```python
from build123d import *

# Parameters (mm, degrees)
SKETCH1_W            = 5
SKETCH1_H            = 4.25
SKETCH2_R            = 2.5
BOSS_EXTRUDE1_DEPTH  = 2.088407645
SKETCH3_R            = 2.5
BOSS_EXTRUDE2_DEPTH  = 0.311592355
BOSS_EXTRUDE2_TAPER  = 55
SKETCH4_R            = 2.055
BOSS_EXTRUDE3_DEPTH  = 0.311592355
BOSS_EXTRUDE3_TAPER  = -55
SKETCH5_R            = 2.5
BOSS_EXTRUDE4_DEPTH  = 0.136815291
SKETCH6_R            = 2.5
BOSS_EXTRUDE5_DEPTH  = 0.311592355
BOSS_EXTRUDE5_TAPER  = 55
SKETCH7_R            = 2.055
BOSS_EXTRUDE6_DEPTH  = 0.311592355
BOSS_EXTRUDE6_TAPER  = -55
SKETCH8_R            = 2.5
BOSS_EXTRUDE7_DEPTH  = 0.136815291
SKETCH9_R            = 2.5
BOSS_EXTRUDE8_DEPTH  = 0.311592355
BOSS_EXTRUDE8_TAPER  = 55
SKETCH10_R           = 2.055
BOSS_EXTRUDE9_DEPTH  = 0.311592355
BOSS_EXTRUDE9_TAPER  = -55
SKETCH11_R           = 2.5
BOSS_EXTRUDE10_DEPTH = 0.136815291
SKETCH12_R           = 2.5
BOSS_EXTRUDE11_DEPTH = 0.311592355
BOSS_EXTRUDE11_TAPER = 55
SKETCH13_R           = 2.055
BOSS_EXTRUDE12_DEPTH = 0.311592355
BOSS_EXTRUDE12_TAPER = -55
SKETCH14_R           = 2.5
BOSS_EXTRUDE13_DEPTH = 0.136815291
SKETCH15_R           = 2.5
BOSS_EXTRUDE14_DEPTH = 0.311592355
BOSS_EXTRUDE14_TAPER = 55
SKETCH16_R           = 2.055
BOSS_EXTRUDE15_DEPTH = 0.311592355
BOSS_EXTRUDE15_TAPER = -55
SKETCH17_R           = 2.5
BOSS_EXTRUDE16_DEPTH = 0.136815291
SKETCH18_R           = 2.5
BOSS_EXTRUDE17_DEPTH = 0.311592355
BOSS_EXTRUDE17_TAPER = 55
SKETCH19_R           = 2.055
BOSS_EXTRUDE18_DEPTH = 0.311592355
BOSS_EXTRUDE18_TAPER = -55
SKETCH20_R           = 2.5
BOSS_EXTRUDE19_DEPTH = 0.136815291
SKETCH21_R           = 2.5
BOSS_EXTRUDE20_DEPTH = 0.311592355
BOSS_EXTRUDE20_TAPER = 55
SKETCH22_R           = 2.055
BOSS_EXTRUDE21_DEPTH = 0.311592355
BOSS_EXTRUDE21_TAPER = -55
SKETCH23_R           = 2.5
BOSS_EXTRUDE22_DEPTH = 0.136815291
SKETCH24_R           = 2.5
BOSS_EXTRUDE23_DEPTH = 0.311592355
BOSS_EXTRUDE23_TAPER = 55
SKETCH25_R           = 2.055
BOSS_EXTRUDE24_DEPTH = 0.311592355
BOSS_EXTRUDE24_TAPER = -55
SKETCH26_R           = 2.5
BOSS_EXTRUDE25_DEPTH = 0.136815291
SKETCH27_R           = 2.5
BOSS_EXTRUDE26_DEPTH = 0.311592355
BOSS_EXTRUDE26_TAPER = 55
SKETCH28_R           = 2.055
BOSS_EXTRUDE27_DEPTH = 0.311592355
BOSS_EXTRUDE27_TAPER = -55
SKETCH29_R           = 2.5
BOSS_EXTRUDE28_DEPTH = 0.136815291
SKETCH30_R           = 2.5
BOSS_EXTRUDE29_DEPTH = 0.311592355
BOSS_EXTRUDE29_TAPER = 55
SKETCH31_R           = 2.055
BOSS_EXTRUDE30_DEPTH = 0.311592355
BOSS_EXTRUDE30_TAPER = -55
SKETCH32_R           = 2.5
BOSS_EXTRUDE31_DEPTH = 0.003407645
SKETCH33_R           = 2.5
BOSS_EXTRUDE32_DEPTH = 0.445
BOSS_EXTRUDE32_TAPER = 45
CUT_EXTRUDE1_DEPTH   = 2.5
FILLET1_R            = 0.2


with BuildPart() as part:
    # Sketch1 → Revolve1 (revolve)
    with BuildSketch(Plane(origin=(0, 0, 0), x_dir=(-1, 0, 0), z_dir=(0, 0, -1))):
        with Locations((6.290592114, 2.355818515)):
            Rectangle(SKETCH1_W, SKETCH1_H)
    revolve(axis=Axis((-3.790592114, 0.230818515, 0), (-1, 0, 0)))

    # Sketch2 → Boss-Extrude1 (add)
    with BuildSketch(Plane(origin=(-3.790592114, 0, 0), x_dir=(0, 0, -1), z_dir=(1, 0, 0))):
        with Locations((0, 0.230818515)):
            Circle(SKETCH2_R)
    extrude(amount=BOSS_EXTRUDE1_DEPTH)

    # Sketch3 → Boss-Extrude2 (add)
    with BuildSketch(Plane(origin=(-1.702184469, 0, 0), x_dir=(0, 0, -1), z_dir=(1, 0, 0))):
        with Locations((0, 0.230818515)):
            Circle(SKETCH3_R)
    extrude(amount=BOSS_EXTRUDE2_DEPTH, taper=BOSS_EXTRUDE2_TAPER)

    # Sketch4 → Boss-Extrude3 (add)
    with BuildSketch(Plane(origin=(-1.390592114, 0, 0), x_dir=(0, 0, -1), z_dir=(1, 0, 0))):
        with Locations((0, 0.230818515)):
            Circle(SKETCH4_R)
    extrude(amount=BOSS_EXTRUDE3_DEPTH, taper=BOSS_EXTRUDE3_TAPER)

    # Sketch5 → Boss-Extrude4 (add)
    with BuildSketch(Plane(origin=(-1.07899976, 0, 0), x_dir=(0, 0, -1), z_dir=(1, 0, 0))):
        with Locations((0, 0.230818515)):
            Circle(SKETCH5_R)
    extrude(amount=BOSS_EXTRUDE4_DEPTH)

    # Sketch6 → Boss-Extrude5 (add)
    with BuildSketch(Plane(origin=(-0.942184469, 0, 0), x_dir=(0, 0, -1), z_dir=(1, 0, 0))):
        with Locations((0, 0.230818515)):
            Circle(SKETCH6_R)
    extrude(amount=BOSS_EXTRUDE5_DEPTH, taper=BOSS_EXTRUDE5_TAPER)

    # Sketch7 → Boss-Extrude6 (add)
    with BuildSketch(Plane(origin=(-0.630592114, 0, 0), x_dir=(0, 0, -1), z_dir=(1, 0, 0))):
        with Locations((0, 0.230818515)):
            Circle(SKETCH7_R)
    extrude(amount=BOSS_EXTRUDE6_DEPTH, taper=BOSS_EXTRUDE6_TAPER)

    # Sketch8 → Boss-Extrude7 (add)
    with BuildSketch(Plane(origin=(-0.31899976, 0, 0), x_dir=(0, 0, -1), z_dir=(1, 0, 0))):
        with Locations((0, 0.230818515)):
            Circle(SKETCH8_R)
    extrude(amount=BOSS_EXTRUDE7_DEPTH)

    # Sketch9 → Boss-Extrude8 (add)
    with BuildSketch(Plane(origin=(-0.182184469, 0, 0), x_dir=(0, 0, -1), z_dir=(1, 0, 0))):
        with Locations((0, 0.230818515)):
            Circle(SKETCH9_R)
    extrude(amount=BOSS_EXTRUDE8_DEPTH, taper=BOSS_EXTRUDE8_TAPER)

    # Sketch10 → Boss-Extrude9 (add)
    with BuildSketch(Plane(origin=(0.129407886, 0, 0), x_dir=(0, 0, -1), z_dir=(1, 0, 0))):
        with Locations((0, 0.230818515)):
            Circle(SKETCH10_R)
    extrude(amount=BOSS_EXTRUDE9_DEPTH, taper=BOSS_EXTRUDE9_TAPER)

    # Sketch11 → Boss-Extrude10 (add)
    with BuildSketch(Plane(origin=(0.44100024, 0, 0), x_dir=(0, 0, -1), z_dir=(1, 0, 0))):
        with Locations((0, 0.230818515)):
            Circle(SKETCH11_R)
    extrude(amount=BOSS_EXTRUDE10_DEPTH)

    # Sketch12 → Boss-Extrude11 (add)
    with BuildSketch(Plane(origin=(0.577815531, 0, 0), x_dir=(0, 0, -1), z_dir=(1, 0, 0))):
        with Locations((0, 0.230818515)):
            Circle(SKETCH12_R)
    extrude(amount=BOSS_EXTRUDE11_DEPTH, taper=BOSS_EXTRUDE11_TAPER)

    # Sketch13 → Boss-Extrude12 (add)
    with BuildSketch(Plane(origin=(0.889407886, 0, 0), x_dir=(0, 0, -1), z_dir=(1, 0, 0))):
        with Locations((0, 0.230818515)):
            Circle(SKETCH13_R)
    extrude(amount=BOSS_EXTRUDE12_DEPTH, taper=BOSS_EXTRUDE12_TAPER)

    # Sketch14 → Boss-Extrude13 (add)
    with BuildSketch(Plane(origin=(1.20100024, 0, 0), x_dir=(0, 0, -1), z_dir=(1, 0, 0))):
        with Locations((0, 0.230818515)):
            Circle(SKETCH14_R)
    extrude(amount=BOSS_EXTRUDE13_DEPTH)

    # Sketch15 → Boss-Extrude14 (add)
    with BuildSketch(Plane(origin=(1.337815531, 0, 0), x_dir=(0, 0, -1), z_dir=(1, 0, 0))):
        with Locations((0, 0.230818515)):
            Circle(SKETCH15_R)
    extrude(amount=BOSS_EXTRUDE14_DEPTH, taper=BOSS_EXTRUDE14_TAPER)

    # Sketch16 → Boss-Extrude15 (add)
    with BuildSketch(Plane(origin=(1.649407886, 0, 0), x_dir=(0, 0, -1), z_dir=(1, 0, 0))):
        with Locations((0, 0.230818515)):
            Circle(SKETCH16_R)
    extrude(amount=BOSS_EXTRUDE15_DEPTH, taper=BOSS_EXTRUDE15_TAPER)

    # Sketch17 → Boss-Extrude16 (add)
    with BuildSketch(Plane(origin=(1.96100024, 0, 0), x_dir=(0, 0, -1), z_dir=(1, 0, 0))):
        with Locations((0, 0.230818515)):
            Circle(SKETCH17_R)
    extrude(amount=BOSS_EXTRUDE16_DEPTH)

    # Sketch18 → Boss-Extrude17 (add)
    with BuildSketch(Plane(origin=(2.097815531, 0, 0), x_dir=(0, 0, -1), z_dir=(1, 0, 0))):
        with Locations((0, 0.230818515)):
            Circle(SKETCH18_R)
    extrude(amount=BOSS_EXTRUDE17_DEPTH, taper=BOSS_EXTRUDE17_TAPER)

    # Sketch19 → Boss-Extrude18 (add)
    with BuildSketch(Plane(origin=(2.409407886, 0, 0), x_dir=(0, 0, -1), z_dir=(1, 0, 0))):
        with Locations((0, 0.230818515)):
            Circle(SKETCH19_R)
    extrude(amount=BOSS_EXTRUDE18_DEPTH, taper=BOSS_EXTRUDE18_TAPER)

    # Sketch20 → Boss-Extrude19 (add)
    with BuildSketch(Plane(origin=(2.72100024, 0, 0), x_dir=(0, 0, -1), z_dir=(1, 0, 0))):
        with Locations((0, 0.230818515)):
            Circle(SKETCH20_R)
    extrude(amount=BOSS_EXTRUDE19_DEPTH)

    # Sketch21 → Boss-Extrude20 (add)
    with BuildSketch(Plane(origin=(2.857815531, 0, 0), x_dir=(0, 0, -1), z_dir=(1, 0, 0))):
        with Locations((0, 0.230818515)):
            Circle(SKETCH21_R)
    extrude(amount=BOSS_EXTRUDE20_DEPTH, taper=BOSS_EXTRUDE20_TAPER)

    # Sketch22 → Boss-Extrude21 (add)
    with BuildSketch(Plane(origin=(3.169407886, 0, 0), x_dir=(0, 0, -1), z_dir=(1, 0, 0))):
        with Locations((0, 0.230818515)):
            Circle(SKETCH22_R)
    extrude(amount=BOSS_EXTRUDE21_DEPTH, taper=BOSS_EXTRUDE21_TAPER)

    # Sketch23 → Boss-Extrude22 (add)
    with BuildSketch(Plane(origin=(3.48100024, 0, 0), x_dir=(0, 0, -1), z_dir=(1, 0, 0))):
        with Locations((0, 0.230818515)):
            Circle(SKETCH23_R)
    extrude(amount=BOSS_EXTRUDE22_DEPTH)

    # Sketch24 → Boss-Extrude23 (add)
    with BuildSketch(Plane(origin=(3.617815531, 0, 0), x_dir=(0, 0, -1), z_dir=(1, 0, 0))):
        with Locations((0, 0.230818515)):
            Circle(SKETCH24_R)
    extrude(amount=BOSS_EXTRUDE23_DEPTH, taper=BOSS_EXTRUDE23_TAPER)

    # Sketch25 → Boss-Extrude24 (add)
    with BuildSketch(Plane(origin=(3.929407886, 0, 0), x_dir=(0, 0, -1), z_dir=(1, 0, 0))):
        with Locations((0, 0.230818515)):
            Circle(SKETCH25_R)
    extrude(amount=BOSS_EXTRUDE24_DEPTH, taper=BOSS_EXTRUDE24_TAPER)

    # Sketch26 → Boss-Extrude25 (add)
    with BuildSketch(Plane(origin=(4.24100024, 0, 0), x_dir=(0, 0, -1), z_dir=(1, 0, 0))):
        with Locations((0, 0.230818515)):
            Circle(SKETCH26_R)
    extrude(amount=BOSS_EXTRUDE25_DEPTH)

    # Sketch27 → Boss-Extrude26 (add)
    with BuildSketch(Plane(origin=(4.377815531, 0, 0), x_dir=(0, 0, -1), z_dir=(1, 0, 0))):
        with Locations((0, 0.230818515)):
            Circle(SKETCH27_R)
    extrude(amount=BOSS_EXTRUDE26_DEPTH, taper=BOSS_EXTRUDE26_TAPER)

    # Sketch28 → Boss-Extrude27 (add)
    with BuildSketch(Plane(origin=(4.689407886, 0, 0), x_dir=(0, 0, -1), z_dir=(1, 0, 0))):
        with Locations((0, 0.230818515)):
            Circle(SKETCH28_R)
    extrude(amount=BOSS_EXTRUDE27_DEPTH, taper=BOSS_EXTRUDE27_TAPER)

    # Sketch29 → Boss-Extrude28 (add)
    with BuildSketch(Plane(origin=(5.00100024, 0, 0), x_dir=(0, 0, -1), z_dir=(1, 0, 0))):
        with Locations((0, 0.230818515)):
            Circle(SKETCH29_R)
    extrude(amount=BOSS_EXTRUDE28_DEPTH)

    # Sketch30 → Boss-Extrude29 (add)
    with BuildSketch(Plane(origin=(5.137815531, 0, 0), x_dir=(0, 0, -1), z_dir=(1, 0, 0))):
        with Locations((0, 0.230818515)):
            Circle(SKETCH30_R)
    extrude(amount=BOSS_EXTRUDE29_DEPTH, taper=BOSS_EXTRUDE29_TAPER)

    # Sketch31 → Boss-Extrude30 (add)
    with BuildSketch(Plane(origin=(5.449407886, 0, 0), x_dir=(0, 0, -1), z_dir=(1, 0, 0))):
        with Locations((0, 0.230818515)):
            Circle(SKETCH31_R)
    extrude(amount=BOSS_EXTRUDE30_DEPTH, taper=BOSS_EXTRUDE30_TAPER)

    # Sketch32 → Boss-Extrude31 (add)
    with BuildSketch(Plane(origin=(5.76100024, 0, 0), x_dir=(0, 0, -1), z_dir=(1, 0, 0))):
        with Locations((0, 0.230818515)):
            Circle(SKETCH32_R)
    extrude(amount=BOSS_EXTRUDE31_DEPTH)

    # Sketch33 → Boss-Extrude32 (add)
    with BuildSketch(Plane(origin=(5.764407886, 0, 0), x_dir=(0, 0, -1), z_dir=(1, 0, 0))):
        with Locations((0, 0.230818515)):
            Circle(SKETCH33_R)
    extrude(amount=BOSS_EXTRUDE32_DEPTH, taper=BOSS_EXTRUDE32_TAPER)

    # Sketch34 → Cut-Extrude1 (cut)
    with BuildSketch(Plane.ZY.offset(8.790592114)):
        Polygon((0, -2.127079985), (2.042, -0.948130735), (2.042, 1.409767764), (0, 2.588717014), (-2.042, 1.409767764), (-2.042, -0.948130735), align=None)
    extrude(amount=-CUT_EXTRUDE1_DEPTH, mode=Mode.SUBTRACT)

    # Sketch35 → Cut-Revolve1 (revolve, cut)
    with BuildSketch(Plane.XY):
        Polygon((-6.290592114, 2.272818515), (-6.290592114, 0.230818515), (-5.111642864, 0.230818515), align=None)
    revolve(axis=Axis((-6.290592114, 0.230818515, 0), (1, 0, 0)), mode=Mode.SUBTRACT)

    # Fillet1
    fillet1_edges = [part.edges().sort_by_distance(p)[0] for p in [
        (-8.790592114, -4.019181485, 0),
        (-3.790592114, 0.230818515, 2.5),
    ]]
    fillet(fillet1_edges, radius=FILLET1_R)


solid = part.part
```
Check sheet for the modelled part. Datum: model origin and axes. Units: mm. Give positions to 0.01 mm unless a question says otherwise; leave off trailing zeros. Write each loop counter-clockwise with the first axis right and the second up, starting at its lowest first coordinate (ties: lowest second). Pieces come first, ordered by that corner, then holes. Notation, with made-up numbers: (8, 46.25) -> (13, 46.25) arc R18 cw to (13, 60.25) -> close; hole circle Ø1 at (77.5, 2). An arc over 180 degrees is marked (long way). Use CSV: the item, a comma, the result in double quotes. Start each with the question number.
Q1. Scan lines: line 1 along X through (y, z) = (-1.75, 2); line 2 along Z through (x, y) = (-7.5, 1.5); line 3 along Y through (x, z) = (-6.5, 0.25). Record each from-to range of solid material in increasing order.
Q2. Release check for a two-part mould opening along Y. For faces 1 (the cylindrical face through (-2.66, -2.21, 0.54)), 2 (the flat face through (-7.558, -1.529, -1.035)) record: +Y half, -Y half, draft (parallel to the pull), parting line (faces both ways), or undercut.
Q3. Cross-section at A-A on x = -4.75. Enter the section's corners in (y, z), and give its area (3 significant figures).
Q4. Cross-section at B-B on x = -2.25. Enter the section's corners in (y, z).
Q5. Depth check by flat-ended pin: P1, Ø1.2, axis at x = -7, y = 0, coming from the +Z side; P2, Ø0.5, axis at y = 1, z = -1.5, coming from the -X side; P3, Ø1, axis at x = -7, z = 2.5, coming from the +Y side; P4, Ø4, axis at x = 0, z = 0.5, coming from the -Y side. Enter the tip coordinate at first touch or a pass-through.
Working result:
1,line 1,"x = -8.79 to -3.79"
1,line 2,"z = -4.06 to -1.89, 1.89 to 4.06"
1,line 3,"y = -4.01 to -1.98, 2.44 to 4.47"
2,face 1,"parting line"
2,face 2,"undercut"
3,outline,"circle Ø8.5 at (0.23, 0)"
3,area,"56.7 mm^2"
4,outline,"circle Ø5 at (0.23, 0)"
5,P1,"stops at z = 4.25"
5,P2,"stops at x = -6.23"
5,P3,"stops at y = 3.98"
5,P4,"stops at y = -2.27"
